Can you work these out from the model? Positions are in its coordinate system, mm. A direction names the side the tool comes from. Give positions to 0.01 mm unless a question says otherwise; leave off trailing zeros. Loops run counter-clockwise (first coordinate to the right, second up) from the corner with the lowest first, then second, coordinate; pieces in that order, holes last. Notation, with made-up numbers: M -17,33 L 20,33 A13 ccw 20,42 Z; hole C 84,-37 d6. An arc over 180 degrees is marked long. One line per item, written item: value. Start each with the question number.
Autodesk Inventor part; units mm, degrees
ref_plane "YZ Plane" through (0, 0, 0) normal (1, 0, 0) x (0, 1, 0)
ref_plane "XZ Plane" through (0, 0, 0) normal (0, 1, 0) x (-1, 0, 0)
ref_plane "XY Plane" through (0, 0, 0) normal (0, 0, 1) x (1, 0, 0)
sketch "Skizze1" plane through (0, 0, 0) normal (0, 0, 1) x (1, 0, 0)
  line L0 (0, 2.8868) -> (2.5, 1.4434)
  line L1 (2.5, 1.4434) -> (2.5, -1.4434)
  line L2 (2.5, -1.4434) -> (0, -2.8868)
  line L3 (0, -2.8868) -> (-2.5, -1.4434)
  line L4 (-2.5, -1.4434) -> (-2.5, 1.4434)
  line L5 (-2.5, 1.4434) -> (0, 2.8868)
  circle A0 centre (0, 0) radius 1.5
  dimension "d0" = 5
  dimension "d1" = 3
extrude "Extrusion1" add sketch "Skizze1" along normal blind 20
chamfer "Fase1" distance 0.3 angle 45 13 edges at (1.25, -2.1651, 20) (-1.25, -2.1651, 20) (2.5, 0, 20) (1.25, 2.1651, 20) (-1.25, 2.1651, 20) (1.25, -2.1651, 0) (2.5, 0, 0) (-1.25, -2.1651, 0) (1.25, 2.1651, 0) (-1.25, 2.1651, 0) (-2.5, 0, 0) (-1.5, 0, 20) (-1.5, 0, 0)
thread "Gewinde1"
sketch "Skizze2" plane through (0, 0, 20) normal (0, 0, 1) x (1, 0, 0)
  line L0 (0, -2.5403) -> (-2.5, -1.097)
  line L1 (2.2, -1.2702) -> (0, -2.5403)
  line L2 (2.2, 1.2702) -> (2.2, -1.2702)
  line L3 (0, 2.5403) -> (2.2, 1.2702)
  line L4 (-2.5, 1.097) -> (0, 2.5403)
  line L5 (-2.5, 1.097) -> (-2.5, -1.097)
  circle A0 centre (0, 0) radius 1.8
extrude "Extrusion2" add sketch "Skizze2" against normal blind 10 contours A0
sketch "Skizze3" plane through (0, 0, 20) normal (0, 0, 1) x (1, 0, 0)
  circle A0 centre (0, 0) radius 1.5
  dimension "d11" = 3
extrude "Extrusion3" add sketch "Skizze3" along normal blind 5
thread "Gewinde2"
chamfer "Fase2" distance 0.3 angle 45 1 edges at (-1.5, 0, 25)
properties part number "Distanzhuelse_M3x20mm_" material "Nickel-Kupfer-Legierung 400"
Q1. If we section it at B-B, the plane y = 0: Write out the boundary of the cut face in (x, z).
Q2. For P1, Ø3, axis at x = 0, y = 2, coming from the +Z side; P2, Ø2, axis at x = 2, z = 19.5, coming from the -Y side; P3, Ø2.5, axis at x = 0.5, y = 0, coming from the -Z side; P4, Ø2.5, axis at x = 0, y = 0, coming from the -Z side, each with a flat end and sliding along its axis, tell me the tip position at first contact or that it passes through.
Q3. If we section it at D-D, the plane z = 23: Write out the boundary of the cut face in (x, y).
Q4. Which directions (+Z, -Z, +X, -X, +Y, -Y) give clear straight access to the entire face, cutting with the end or side of a thin tool? Please do faces 1 (the face through (-1.5, -0.07, 22.32)), 2 (the face through (2.5, 0, 10)), 3 (the face through (-1.5, -0.07, 5.08)).
Q5. If we section it at C-C, the plane z = 10.25: Write out the boundary of the cut face in (x, y).
Q6. I need wall thicknesses on line 1 along X through (y, z) = (0, 7.75); line 2 along X through (y, z) = (-0.8, 4); line 3 along Z through (x, y) = (-1.8, -0.9). Which ranges of each line are inside material? Lowest first, please.
Q7. If we section it at A-A, the plane z = 2.75: Write out the boundary of the cut face in (x, y).
Q8. If we mould it in two halves opening along Y, with no side actions, what happens to faces 4 (the face through (-1.156, 2.043, 0.148)), 5 (the face through (0, 0, 10)), 6 (the face through (1.267, -2.155, 9.864))? For each: released by +Y, released by -Y, zero draft, split by the parting line, or undercut.
Response:
1. outline: M -2.5,0.3 L -2.2,0 L -1.8,0 L -1.5,0.3 L -1.5,10 L 1.5,10 L 1.5,0.3 L 1.8,0 L 2.2,0 L 2.5,0.3 L 2.5,19.7 L 2.2,20 L 1.5,20 L 1.5,24.7 L 1.2,25 L -1.2,25 L -1.5,24.7 L -1.5,20 L -2.5,20 Z
2. P1: z = 25
2. P2: y = -2.31
2. P3: z = 0.05
2. P4: z = 10
3. outline: C 0,0 d3
4. face 1: +Z
4. face 2: +Z, -Z, +X, +Y, -Y
4. face 3: -Z
5. outline: M -2.5,-1.44 L 0,-2.89 L 2.5,-1.44 L 2.5,1.44 L 0,2.89 L -2.5,1.44 Z
6. line 1: -2.5 to -1.5, 1.5 to 2.5
6. line 2: -2.5 to -1.27, 1.27 to 2.5
6. line 3: 0 to 20
7. outline: M -2.5,-1.44 L 0,-2.89 L 2.5,-1.44 L 2.5,1.44 L 0,2.89 L -2.5,1.44 Z; hole C 0,0 d3
8. face 4: released by +Y
8. face 5: undercut
8. face 6: released by -Y
